CAD build for the part. Positions are in the model's coordinates, mm. Give positions to 0.01 mm unless a question says otherwise; leave off trailing zeros. Write each loop counter-clockwise with the first axis right and the second up, starting at its lowest first coordinate (ties: lowest second). Pieces come first, ordered by that corner, then holes. Notation, with made-up numbers: (-4, 86) - (20, 86) arc R16 ccw to (20, 109) - close; hole circle Ø8 at (13.25, 53). An arc over 180 degrees is marked (long way). Put each result on its own line as item: value. Start each with the question number.
1. Drop flat-ended pins along their axis: pin 1 (5 mm diameter, centred on x = -66, z = 80.5, fed in from -Y); pin 2 (5 mm diameter, centred on x = -109.5, z = -7, fed in from -Y); pin 3 (8 mm diameter, centred on x = -259, y = 148.5, fed in from +Z). Give the stop position or say it passes through.
2. Wall check: line 1 (Z direction, x = -340, y = -32); line 2 (X direction, y = -869.5, z = -2.5). Give the ranges that are in metal, low to high.
3. Cut at D-D on y = -259.5. List the corners of the cut face in (x, z), and give its area (3 significant figures).
4. Cut at C-C on x = -539.5. List the corners of the cut face in (y, z).
5. Cut at A-A on y = -848. List the corners of the cut face in (x, z).
6. Cut at B-B on x = -109.5. List the corners of the cut face in (y, z).
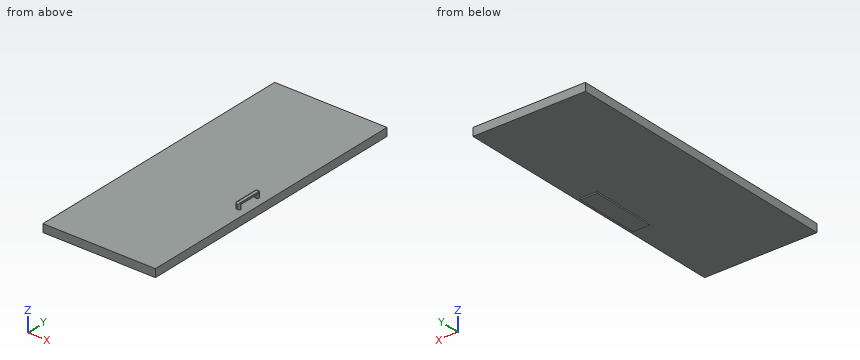
from build123d import *

# Parameters (mm, degrees)
BOSS_EXTRUDE2_DEPTH = 57.15
BOSS_EXTRUDE3_DEPTH = 44
CUT_EXTRUDE1_DEPTH  = 44
FILLET1_R           = 10
SKETCH6_W           = 120
SKETCH6_H           = 460.0000000000001
BOSS_EXTRUDE4_DEPTH = 10


with BuildPart() as part:
    # Sketch1 → Boss-Extrude2 (new body)
    with BuildSketch(Plane.XY):
        Polygon((0, 0), (0, 446.2018372120283), (-800, 446.2018372120282), (-799.9999999999998, -1585.7981627879717), (0, -1585.7981627879717), align=None)
    extrude(amount=BOSS_EXTRUDE2_DEPTH)

    # Sketch4 → Boss-Extrude3 (add)
    with BuildSketch(Plane.XY.offset(57.15)):
        Polygon((-79.99999999999993, -603.7981627879718), (-49.999999999999936, -603.7981627879718), (-49.999999999999915, -785.7981627879718), (-79.9999999999999, -785.7981627879718), align=None)
    extrude(amount=BOSS_EXTRUDE3_DEPTH)

    # Sketch5 → Cut-Extrude1 (cut)
    with BuildSketch(Plane.ZY.offset(80.00000000000003)):
        Polygon((83.14999999999999, -624.7981627879717), (57.150000000000006, -624.7981627879717), (57.15, -764.7981627879717), (83.15, -764.7981627879717), align=None)
    extrude(amount=-CUT_EXTRUDE1_DEPTH, mode=Mode.SUBTRACT)

    # Fillet1
    # the kernel refuses this fillet: 10 mm, written as the material it takes off along each edge
    with BuildSketch(Plane(origin=(-69.99999999999993, -613.7981627879718, 91.15), x_dir=(-1, -1.6e-16, 0), z_dir=(0, 1, 0))) as fillet1_piece_1_section:
        Polygon((0, 0), (FILLET1_R, 0), (FILLET1_R, FILLET1_R), (0, FILLET1_R), align=None)
    fillet1_piece_1 = extrude(amount=FILLET1_R, mode=Mode.PRIVATE)
    fillet1_piece_1 = fillet1_piece_1 - Plane(origin=(-69.99999999999993, -613.7981627879718, 91.15), x_dir=(0.7071067811865475, 0, -0.7071067811865475), z_dir=(0, 1, 0)) * Sphere(FILLET1_R, mode=Mode.PRIVATE)
    add(fillet1_piece_1, mode=Mode.SUBTRACT)
    with BuildSketch(Plane(origin=(-69.9999999999999, -775.7981627879718, 91.15), x_dir=(0, 0, 1), z_dir=(-1, -1.6e-16, 0))) as fillet1_piece_2_section:
        Polygon((0, 0), (FILLET1_R, 0), (FILLET1_R, -FILLET1_R), (0, -FILLET1_R), align=None)
    fillet1_piece_2 = extrude(amount=FILLET1_R, mode=Mode.PRIVATE)
    fillet1_piece_2 = fillet1_piece_2 - Plane(origin=(-69.9999999999999, -775.7981627879718, 91.15), x_dir=(0, 0.7071067811865475, -0.7071067811865475), z_dir=(-1, -1.6e-16, 0)) * Sphere(FILLET1_R, mode=Mode.PRIVATE)
    add(fillet1_piece_2, mode=Mode.SUBTRACT)
    with BuildSketch(Plane(origin=(-49.999999999999915, -785.7981627879718, 57.15), x_dir=(-1, 0, 0), z_dir=(0, 0, 1))) as fillet1_piece_3:
        with BuildLine():
            CenterArc((FILLET1_R, -FILLET1_R), FILLET1_R, 90, 90)
            Line((0, -FILLET1_R), (0, 0))
            Line((0, 0), (FILLET1_R, 0))
        make_face()
    extrude(amount=69, mode=Mode.SUBTRACT)
    with BuildSketch(Plane(origin=(-49.999999999999936, -603.7981627879718, 57.15), x_dir=(0, -1, 0), z_dir=(0, 0, 1))) as fillet1_piece_4:
        with BuildLine():
            CenterArc((FILLET1_R, -FILLET1_R), FILLET1_R, 90, 90)
            Line((0, -FILLET1_R), (0, 0))
            Line((0, 0), (FILLET1_R, 0))
        make_face()
    extrude(amount=69, mode=Mode.SUBTRACT)
    with BuildSketch(Plane(origin=(-79.99999999999993, -603.7981627879718, 57.15), x_dir=(1, 0, 0), z_dir=(0, 0, 1))) as fillet1_piece_5:
        with BuildLine():
            CenterArc((FILLET1_R, -FILLET1_R), FILLET1_R, 90, 90)
            Line((0, -FILLET1_R), (0, 0))
            Line((0, 0), (FILLET1_R, 0))
        make_face()
    extrude(amount=34.00000000000001, mode=Mode.SUBTRACT)
    with BuildSketch(Plane(origin=(-79.9999999999999, -785.7981627879718, 57.15), x_dir=(1, 0, 0), z_dir=(0, 0, 1))) as fillet1_piece_6:
        with BuildLine():
            CenterArc((FILLET1_R, FILLET1_R), FILLET1_R, 180, 90)
            Line((0, FILLET1_R), (0, 0))
            Line((0, 0), (FILLET1_R, 0))
        make_face()
    extrude(amount=34.00000000000001, mode=Mode.SUBTRACT)
    with BuildSketch(Plane(origin=(-69.99999999999993, -603.7981627879718, 101.15), x_dir=(0, 0, -1), z_dir=(1, 0, 0))) as fillet1_piece_7:
        with BuildLine():
            CenterArc((FILLET1_R, -FILLET1_R), FILLET1_R, 90, 90)
            Line((0, -FILLET1_R), (0, 0))
            Line((0, 0), (FILLET1_R, 0))
        make_face()
    extrude(amount=44.99999999999999, mode=Mode.SUBTRACT)
    with BuildSketch(Plane(origin=(-79.9999999999999, -775.7981627879718, 101.15), x_dir=(0, 0, -1), z_dir=(-1.6e-16, 1, 0))) as fillet1_piece_8:
        with BuildLine():
            CenterArc((FILLET1_R, -FILLET1_R), FILLET1_R, 90, 90)
            Line((0, -FILLET1_R), (0, 0))
            Line((0, 0), (FILLET1_R, 0))
        make_face()
    extrude(amount=162, mode=Mode.SUBTRACT)
    with BuildSketch(Plane(origin=(-24.999999999999915, -785.7981627879718, 101.15), x_dir=(0, 0, -1), z_dir=(-1, 0, 0))) as fillet1_piece_9:
        with BuildLine():
            CenterArc((FILLET1_R, -FILLET1_R), FILLET1_R, 90, 90)
            Line((0, -FILLET1_R), (0, 0))
            Line((0, 0), (FILLET1_R, 0))
        make_face()
    extrude(amount=44.999999999999986, mode=Mode.SUBTRACT)
    with BuildSketch(Plane(origin=(-79.99999999999991, -764.7981627879717, 57.15000000000002), x_dir=(1.42e-15, -1, 0), z_dir=(0, 0, 1))) as fillet1_piece_10:
        with BuildLine():
            CenterArc((FILLET1_R, FILLET1_R), FILLET1_R, 180, 89.99999999999989)
            Line((1.421e-14, FILLET1_R), (0, 0))
            Line((0, 0), (FILLET1_R, 0))
        make_face()
    extrude(amount=25.999999999999986, mode=Mode.SUBTRACT)
    with BuildSketch(Plane(origin=(-79.99999999999993, -624.7981627879717, 83.14999999999999), x_dir=(0, 1, 0), z_dir=(0, 0, -1))) as fillet1_piece_11:
        with BuildLine():
            CenterArc((FILLET1_R, FILLET1_R), FILLET1_R, 180, 90)
            Line((0, FILLET1_R), (0, 0))
            Line((0, 0), (FILLET1_R, 0))
        make_face()
    extrude(amount=25.999999999999986, mode=Mode.SUBTRACT)
    with BuildSketch(Plane(origin=(-79.99999999999991, -764.7981627879717, 83.15), x_dir=(1.42e-15, 1e-16, 1), z_dir=(-1.5e-16, 1, -1e-16))) as fillet1_piece_12:
        with BuildLine():
            CenterArc((FILLET1_R, FILLET1_R), FILLET1_R, 180, 89.99999999999989)
            Line((1.421e-14, FILLET1_R), (0, 0))
            Line((0, 0), (FILLET1_R, 0))
        make_face()
    extrude(amount=140, mode=Mode.SUBTRACT)
    with BuildSketch(Plane(origin=(-49.999999999999915, -764.7981627879717, 83.15), x_dir=(0, -1, 0), z_dir=(0, 0, -1))) as fillet1_piece_13:
        with BuildLine():
            CenterArc((FILLET1_R, FILLET1_R), FILLET1_R, 180, 90)
            Line((0, FILLET1_R), (0, 0))
            Line((0, 0), (FILLET1_R, 0))
        make_face()
    extrude(amount=26, mode=Mode.SUBTRACT)
    with BuildSketch(Plane(origin=(-49.999999999999936, -624.7981627879717, 57.150000000000006), x_dir=(0, 1, 0), z_dir=(0, 0, 1))) as fillet1_piece_14:
        with BuildLine():
            CenterArc((FILLET1_R, FILLET1_R), FILLET1_R, 180.00000000000003, 90)
            Line((0, FILLET1_R), (0, 0))
            Line((0, 0), (FILLET1_R, 0))
        make_face()
    extrude(amount=25.999999999999986, mode=Mode.SUBTRACT)
    with BuildSketch(Plane(origin=(-49.999999999999936, -624.7981627879717, 83.15), x_dir=(0, 1e-16, 1), z_dir=(1.2e-16, -1, 1e-16))) as fillet1_piece_15:
        with BuildLine():
            CenterArc((FILLET1_R, FILLET1_R), FILLET1_R, 180, 90)
            Line((0, FILLET1_R), (0, 0))
            Line((0, 0), (FILLET1_R, 0))
        make_face()
    extrude(amount=140, mode=Mode.SUBTRACT)
    with BuildSketch(Plane(origin=(-79.99999999999991, -764.7981627879717, 57.15000000000002), x_dir=(1.42e-15, -1, 0), z_dir=(0, 0, 1))) as fillet1_piece_16a_section:
        with BuildLine():
            CenterArc((FILLET1_R, FILLET1_R), FILLET1_R, 180, 89.99999999999989)
            Line((1.421e-14, FILLET1_R), (0, 0))
            Line((0, 0), (FILLET1_R, 0))
        make_face()
    fillet1_piece_16a = extrude(amount=50.999999999999986, mode=Mode.PRIVATE)
    fillet1_piece_16a = split(fillet1_piece_16a, bisect_by=Plane(origin=(-77.7360488573316, -767.0621139306398, 83.15), z_dir=(0, 1e-16, 1)), keep=Keep.TOP, mode=Mode.PRIVATE)
    with BuildSketch(Plane(origin=(-79.9999999999999, -789.7981627879717, 83.15), x_dir=(0, 1e-16, 1), z_dir=(-1.5e-16, 1, -1e-16))) as fillet1_piece_16b_section:
        with BuildLine():
            CenterArc((FILLET1_R, FILLET1_R), FILLET1_R, 180, 90)
            Line((0, FILLET1_R), (0, 0))
            Line((0, 0), (FILLET1_R, 0))
        make_face()
    fillet1_piece_16b = extrude(amount=165, mode=Mode.PRIVATE)
    fillet1_piece_16b = split(fillet1_piece_16b, bisect_by=Plane(origin=(-77.73604885733165, -764.7981627879717, 85.41395114266827), z_dir=(1.5e-16, -1, 0)), keep=Keep.TOP, mode=Mode.PRIVATE)
    fillet1_piece_16 = fillet1_piece_16a & fillet1_piece_16b
    add(fillet1_piece_16, mode=Mode.SUBTRACT)
    with BuildSketch(Plane(origin=(-79.99999999999991, -764.7981627879717, 83.15), x_dir=(1.42e-15, 1e-16, 1), z_dir=(-1.5e-16, 1, -1e-16))) as fillet1_piece_17a_section:
        with BuildLine():
            CenterArc((FILLET1_R, FILLET1_R), FILLET1_R, 180, 89.99999999999989)
            Line((1.421e-14, FILLET1_R), (0, 0))
            Line((0, 0), (FILLET1_R, 0))
        make_face()
    fillet1_piece_17a = extrude(amount=165, mode=Mode.PRIVATE)
    fillet1_piece_17a = split(fillet1_piece_17a, bisect_by=Plane(origin=(-77.73604885733167, -624.7981627879717, 85.41395114266825), z_dir=(-1.5e-16, 1, 0)), keep=Keep.TOP, mode=Mode.PRIVATE)
    with BuildSketch(Plane(origin=(-79.99999999999993, -624.7981627879717, 108.14999999999998), x_dir=(0, 1, 0), z_dir=(0, 0, -1))) as fillet1_piece_17b_section:
        with BuildLine():
            CenterArc((FILLET1_R, FILLET1_R), FILLET1_R, 180, 90)
            Line((0, FILLET1_R), (0, 0))
            Line((0, 0), (FILLET1_R, 0))
        make_face()
    fillet1_piece_17b = extrude(amount=50.999999999999986, mode=Mode.PRIVATE)
    fillet1_piece_17b = split(fillet1_piece_17b, bisect_by=Plane(origin=(-77.73604885733164, -622.5342116453035, 83.14999999999999), z_dir=(0, 1e-16, 1)), keep=Keep.TOP, mode=Mode.PRIVATE)
    fillet1_piece_17 = fillet1_piece_17a & fillet1_piece_17b
    add(fillet1_piece_17, mode=Mode.SUBTRACT)
    with BuildSketch(Plane(origin=(-49.999999999999936, -624.7981627879717, 83.15), x_dir=(0, 1e-16, 1), z_dir=(1.2e-16, -1, 1e-16))) as fillet1_piece_18a_section:
        with BuildLine():
            CenterArc((FILLET1_R, FILLET1_R), FILLET1_R, 180, 90)
            Line((0, FILLET1_R), (0, 0))
            Line((0, 0), (FILLET1_R, 0))
        make_face()
    fillet1_piece_18a = extrude(amount=165, mode=Mode.PRIVATE)
    fillet1_piece_18a = split(fillet1_piece_18a, bisect_by=Plane(origin=(-52.26395114266817, -764.7981627879717, 85.41395114266827), z_dir=(1.5e-16, -1, 0)), keep=Keep.TOP, mode=Mode.PRIVATE)
    with BuildSketch(Plane(origin=(-49.999999999999915, -764.7981627879717, 108.15), x_dir=(0, -1, 0), z_dir=(0, 0, -1))) as fillet1_piece_18b_section:
        with BuildLine():
            CenterArc((FILLET1_R, FILLET1_R), FILLET1_R, 180, 90)
            Line((0, FILLET1_R), (0, 0))
            Line((0, 0), (FILLET1_R, 0))
        make_face()
    fillet1_piece_18b = extrude(amount=51, mode=Mode.PRIVATE)
    fillet1_piece_18b = split(fillet1_piece_18b, bisect_by=Plane(origin=(-52.2639511426682, -767.0621139306397, 83.15), z_dir=(0, 1e-16, 1)), keep=Keep.TOP, mode=Mode.PRIVATE)
    fillet1_piece_18 = fillet1_piece_18a & fillet1_piece_18b
    add(fillet1_piece_18, mode=Mode.SUBTRACT)
    with BuildSketch(Plane(origin=(-49.999999999999936, -624.7981627879717, 57.150000000000006), x_dir=(0, 1, 0), z_dir=(0, 0, 1))) as fillet1_piece_19a_section:
        with BuildLine():
            CenterArc((FILLET1_R, FILLET1_R), FILLET1_R, 180.00000000000003, 90)
            Line((0, FILLET1_R), (0, 0))
            Line((0, 0), (FILLET1_R, 0))
        make_face()
    fillet1_piece_19a = extrude(amount=50.999999999999986, mode=Mode.PRIVATE)
    fillet1_piece_19a = split(fillet1_piece_19a, bisect_by=Plane(origin=(-52.26395114266823, -622.5342116453035, 83.14999999999999), z_dir=(0, 1e-16, 1)), keep=Keep.TOP, mode=Mode.PRIVATE)
    with BuildSketch(Plane(origin=(-49.999999999999936, -599.7981627879717, 83.14999999999999), x_dir=(0, 1e-16, 1), z_dir=(1.2e-16, -1, 1e-16))) as fillet1_piece_19b_section:
        with BuildLine():
            CenterArc((FILLET1_R, FILLET1_R), FILLET1_R, 179.99999999999997, 90)
            Line((0, FILLET1_R), (0, 0))
            Line((0, 0), (FILLET1_R, 0))
        make_face()
    fillet1_piece_19b = extrude(amount=165, mode=Mode.PRIVATE)
    fillet1_piece_19b = split(fillet1_piece_19b, bisect_by=Plane(origin=(-52.26395114266818, -624.7981627879717, 85.41395114266824), z_dir=(-1.5e-16, 1, 0)), keep=Keep.TOP, mode=Mode.PRIVATE)
    fillet1_piece_19 = fillet1_piece_19a & fillet1_piece_19b
    add(fillet1_piece_19, mode=Mode.SUBTRACT)

    # Sketch6 → Boss-Extrude4 (add)
    with BuildSketch(Plane(origin=(0, 0, 0), x_dir=(-1, 0, 0), z_dir=(0, 0, -1))):
        with Locations((85, -694.7981627879719)):
            Rectangle(SKETCH6_W, SKETCH6_H)
    extrude(amount=BOSS_EXTRUDE4_DEPTH)


solid = part.part
Report:
1. pin 1: stops at y = -785.8
1. pin 2: stops at y = -924.8
1. pin 3: stops at z = 57.15
2. line 1: z = 0 to 57.15
2. line 2: x = -145 to -25
3. outline: (-800, 0) - (0, 0) - (0, 57.15) - (-800, 57.15) - close
3. area: 45,700 mm²
4. outline: (-1585.8, 0) - (446.2, 0) - (446.2, 57.15) - (-1585.8, 57.15) - close
5. outline: (-800, 0) - (-145, 0) - (-145, -10) - (-25, -10) - (-25, 0) - (0, 0) - (0, 57.15) - (-800, 57.15) - close
6. outline: (-1585.8, 0) - (-924.8, 0) - (-924.8, -10) - (-464.8, -10) - (-464.8, 0) - (446.2, 0) - (446.2, 57.15) - (-1585.8, 57.15) - close
